```python
from build123d import *

# Parameters (mm, degrees)
SKETCH1_W           = 8.5
SKETCH1_H           = 10.5
BOSS_EXTRUDE1_DEPTH = 12.5
SKETCH2_W           = 8.5
SKETCH2_H           = 2
CUT_EXTRUDE1_DEPTH  = 8
BOSS_EXTRUDE2_DEPTH = 2
CHAMFER1_SIZE       = 1


with BuildPart() as part:
    # Sketch1 → Boss-Extrude1 (new body)
    with BuildSketch(Plane.XY):
        Rectangle(SKETCH1_W, SKETCH1_H)
    extrude(amount=BOSS_EXTRUDE1_DEPTH)

    # Sketch2 → Cut-Extrude1 (cut)
    with BuildSketch(Plane.XY.offset(12.5)):
        with Locations((0, -0.25)):
            Rectangle(SKETCH2_W, SKETCH2_H)
    extrude(amount=-CUT_EXTRUDE1_DEPTH, mode=Mode.SUBTRACT)

    # Sketch3 → Boss-Extrude2 (add)
    # profile 1 of 2: a face of its own
    with BuildSketch(Plane.XZ.offset(5.25)):
        with BuildLine():
            Line((4.25, 0), (8, 0))
            ThreePointArc((8, 0), (9.414213562, 0.585786438), (10, 2))
            Line((10, 2), (10, 5))
            ThreePointArc((10, 5), (9.414213562, 6.414213562), (8, 7))
            Line((8, 7), (4.25, 7))
            Line((4.25, 7), (4.25, 0))
        make_face()
        with BuildLine():
            Line((6, 2.5), (6, 3.5))
            ThreePointArc((6, 3.5), (7.5, 5), (9, 3.5))
            Line((9, 3.5), (9, 2.5))
            ThreePointArc((9, 2.5), (7.5, 1), (6, 2.5))
        make_face(mode=Mode.SUBTRACT)
    # profile 2 of 2: a face of its own
    with BuildSketch(Plane.XZ.offset(5.25)):
        with BuildLine():
            Line((-10, 2), (-10, 5))
            ThreePointArc((-10, 5), (-9.414213562, 6.414213562), (-8, 7))
            Line((-8, 7), (-4.25, 7))
            Line((-4.25, 7), (-4.25, 0))
            Line((-4.25, 0), (-8, 0))
            ThreePointArc((-8, 0), (-9.414213562, 0.585786438), (-10, 2))
        make_face()
        with BuildLine():
            Line((-6, 2.5), (-6, 3.5))
            ThreePointArc((-6, 3.5), (-7.5, 5), (-9, 3.5))
            Line((-9, 3.5), (-9, 2.5))
            ThreePointArc((-9, 2.5), (-7.5, 1), (-6, 2.5))
        make_face(mode=Mode.SUBTRACT)
    extrude(amount=-BOSS_EXTRUDE2_DEPTH)

    # Chamfer1
    chamfer1_edges = [part.edges().sort_by_distance(p)[0] for p in [
        (-4.25, 3, 12.5),
        (4.25, 3, 12.5),
        (-4.25, -3.25, 12.5),
        (4.25, -3.25, 12.5),
    ]]
    chamfer(chamfer1_edges, length=CHAMFER1_SIZE)


solid = part.part
```
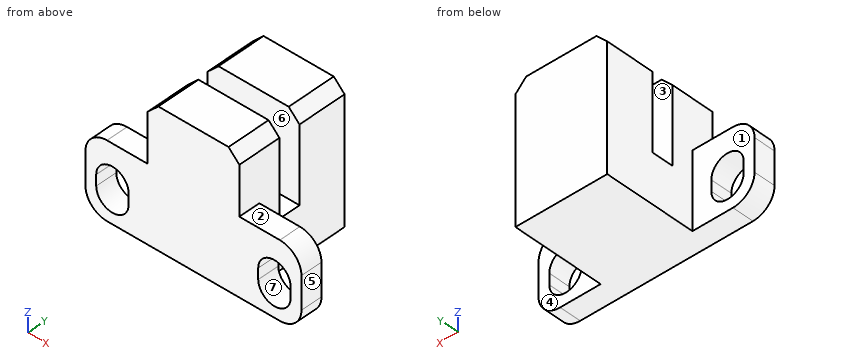
Input: part model. Units: mm. Frame: model coordinates. Face numbers are marked on the shaded views. A direction names the side the tool comes from. Round coordinates to 2 decimals unless told otherwise and drop trailing zeros. Loops run counter-clockwise (first coordinate to the right, second up) from the corner with the lowest first, then second, coordinate; pieces in that order, holes last. Notation, with made-up numbers: (9.25, 84) -> (22.25, 84) arc R35 ccw to (22.25, 123) -> close; hole circle Ø4 at (67, 10.25). An arc over 180 degrees is marked (long way). Use one line per item in the form item = value. Start each with the question number.
Item 1: Mould query, pull axis X, two halves, no side actions, for the marked faces 5, 6 and 7. Classes: pulls with the +X half, pulls with the -X half, needs draft (parallel to the pull), parting line crosses it, or undercut.
Item 2: Set-up query: the marked faces 1, 2, 3 and 4. Return all of +Z, -Z, +X, -X, +Y, -Y with unobstructed straight access to the full face (end or side cutting, diameter ignored); none if empty.
Item 3: Section query C-C on y = -4. Return the cut outline in (x, z).
Item 4: Section query B-B on z = 2.75. Return the cut outline in (x, y).
Item 5: Section query A-A on x = 7.5. Return the cut outline in (y, z).
Item 6: Material intervals for L1, parallel to Y at x = 3.5, z = 4.75; L2, parallel to Y at x = 6, z = 1.75; L3, parallel to Z at x = -0.5, y = 0.5, sorted ascending. Write a range as from..to.
Item 7: Section query D-D on z = 10.5. Return the cut outline in (x, y).
Item 8: Contact query for flat-ended pins moving along their axis: pin 1 Ø3 at (y, z) = (2.5, 6) entering from -X; pin 2 Ø4.5 at (x, z) = (7, 5) entering from +Y; pin 3 Ø1 at (x, y) = (1, -0.5) entering from +Z. Output: stop coordinate, or through.
Ans:
q1.face_5 = pulls with the +X half
q1.face_6 = needs draft
q1.face_7 = undercut
q2.face_1 = +Z, -Z, -X, +Y
q2.face_2 = +Z, +X, +Y, -Y
q2.face_3 = +Z, +X, -X
q2.face_4 = +Z, -Z, +X, +Y
q3.outline = (-10, 2) arc R2 ccw to (-8, 0) -> (8, 0) arc R2 ccw to (10, 2) -> (10, 5) arc R2 ccw to (8, 7) -> (4.25, 7) -> (4.25, 11.5) -> (3.25, 12.5) -> (-3.25, 12.5) -> (-4.25, 11.5) -> (-4.25, 7) -> (-8, 7) arc R2 ccw to (-10, 5) -> close; hole (-9, 2.5) arc R1.5 ccw to (-6, 2.5) -> (-6, 3.5) arc R1.5 ccw to (-9, 3.5) -> close; hole (6, 2.5) arc R1.5 ccw to (9, 2.5) -> (9, 3.5) arc R1.5 ccw to (6, 3.5) -> close
q4.outline = (-10, -5.25) -> (-9, -5.25) -> (-9, -3.25) -> (-10, -3.25) -> close; (-6, -5.25) -> (6, -5.25) -> (6, -3.25) -> (4.25, -3.25) -> (4.25, 5.25) -> (-4.25, 5.25) -> (-4.25, -3.25) -> (-6, -3.25) -> close; (9, -5.25) -> (10, -5.25) -> (10, -3.25) -> (9, -3.25) -> close
q5.outline = (-5.25, 0) -> (-3.25, 0) -> (-3.25, 1) -> (-5.25, 1) -> close; (-5.25, 5) -> (-3.25, 5) -> (-3.25, 7) -> (-5.25, 7) -> close
q6.L1 = -5.25..-1.25, 0.75..5.25
q6.L2 = -5.25..-3.25
q6.L3 = 0..4.5
q7.outline = (-4.25, -5.25) -> (4.25, -5.25) -> (4.25, -1.25) -> (-4.25, -1.25) -> close; (-4.25, 0.75) -> (4.25, 0.75) -> (4.25, 5.25) -> (-4.25, 5.25) -> close
q8.pin_1 = -4.25
q8.pin_2 = -3.25
q8.pin_3 = 4.5
